Design review of the part built by this model. Coordinates are the model's own, in mm. Face numbers are marked on the shaded views. A direction names the side the tool comes from. Coordinates: 2 decimals unless noted, no trailing zeros. Write each loop counter-clockwise with the first axis right and the second up, starting at its lowest first coordinate (ties: lowest second). Pieces come first, ordered by that corner, then holes. Notation, with made-up numbers: (45, 1.5) -> (95, 1.5) arc R27 ccw to (95, 19.5) -> close; hole circle Ø4 at (43, 29). An arc over 180 degrees is marked (long way). Return JSON: item names as keys, results as strings. Group by question number.
from build123d import *

# Parameters (mm, degrees)
SKETCH_3_W          = 280
SKETCH_3_H          = 100
EXTRUDE_1_DEPTH     = 10
SKETCH_5_R          = 4
CUT_EXTRUDE_1_DEPTH = 149.996644258
SKETCH_6_R          = 4
CUT_EXTRUDE_2_DEPTH = 10
SKETCH_7_W          = 50
SKETCH_7_H          = 40
CUT_EXTRUDE_3_DEPTH = 149.996644258
FILLET_1_R          = 10
FILLET_2_R          = 10
SKETCH_8_W          = 40
SKETCH_8_H          = 40
CUT_EXTRUDE_4_DEPTH = 149.996644258
SKETCH_11_R         = 11
CUT_EXTRUDE_5_DEPTH = 5


with BuildPart() as part:
    # 草图3 → 凸台-拉伸1 (new body)
    with BuildSketch(Plane(origin=(0, 0, 0), x_dir=(1, 0, 0), z_dir=(0, 1, 0))):
        Rectangle(SKETCH_3_W, SKETCH_3_H)
    extrude(amount=EXTRUDE_1_DEPTH)

    # 草图5 → 切除-拉伸1 (cut, through all)
    with BuildSketch(Plane(origin=(0, 10, 0), x_dir=(1, 0, 0), z_dir=(0, 1, 0))):
        with Locations(Location((-115, -30, 0), (0, 0, 270))):
            Circle(SKETCH_5_R)
        with Locations(Location((-90, -30, 0), (0, 0, 270))):
            Circle(SKETCH_5_R)
    cut_extrude_1 = extrude(amount=-CUT_EXTRUDE_1_DEPTH, mode=Mode.SUBTRACT)

    # 镜向1: 切除-拉伸1 across plane
    add(cut_extrude_1.mirror(Plane.XY), mode=Mode.SUBTRACT)

    # 草图6 → 切除-拉伸2 (cut)
    with BuildSketch(Plane(origin=(0, 10, 0), x_dir=(1, 0, 0), z_dir=(0, 1, 0))):
        with Locations(Location((125, 30, 0), (0, 0, 270))):
            Circle(SKETCH_6_R)
        with Locations(Location((100, 30, 0), (0, 0, 270))):
            Circle(SKETCH_6_R)
    cut_extrude_2 = extrude(amount=-CUT_EXTRUDE_2_DEPTH, mode=Mode.SUBTRACT)

    # 镜向2: 切除-拉伸2 across plane
    add(cut_extrude_2.mirror(Plane.XY), mode=Mode.SUBTRACT)

    # 草图7 → 切除-拉伸3 (cut, through all)
    with BuildSketch(Plane(origin=(0, 10, 0), x_dir=(1, 0, 0), z_dir=(0, 1, 0))):
        with Locations((-115, 0)):
            Rectangle(SKETCH_7_W, SKETCH_7_H)
    extrude(amount=-CUT_EXTRUDE_3_DEPTH, mode=Mode.SUBTRACT)

    # 圆角1
    fillet_1_edges = [part.edges().sort_by_distance(p)[0] for p in [
        (-140, 5, 50),
    ]]
    fillet(fillet_1_edges, radius=FILLET_1_R)

    # 圆角2
    fillet_2_edges = [part.edges().sort_by_distance(p)[0] for p in [
        (-140, 5, -50),
    ]]
    fillet(fillet_2_edges, radius=FILLET_2_R)

    # 草图8 → 切除-拉伸4 (cut, through all)
    with BuildSketch(Plane(origin=(0, 10, 0), x_dir=(1, 0, 0), z_dir=(0, 1, 0))):
        with Locations((120, 0)):
            Rectangle(SKETCH_8_W, SKETCH_8_H)
    extrude(amount=-CUT_EXTRUDE_4_DEPTH, mode=Mode.SUBTRACT)

    # 草图11 → 切除-拉伸5 (cut)
    with BuildSketch(Plane(origin=(0, 10, 0), x_dir=(1, 0, 0), z_dir=(0, 1, 0))):
        with Locations(Location((-69.5, -34.5, 0), (0, 0, 270))):
            Circle(SKETCH_11_R)
        with Locations(Location((-69.5, 34.5, 0), (0, 0, 270))):
            Circle(SKETCH_11_R)
        with Locations(Location((69.5, 34.5, 0), (0, 0, 270))):
            Circle(SKETCH_11_R)
        with Locations(Location((69.5, -34.5, 0), (0, 0, 270))):
            Circle(SKETCH_11_R)
    extrude(amount=-CUT_EXTRUDE_5_DEPTH, mode=Mode.SUBTRACT)


solid = part.part
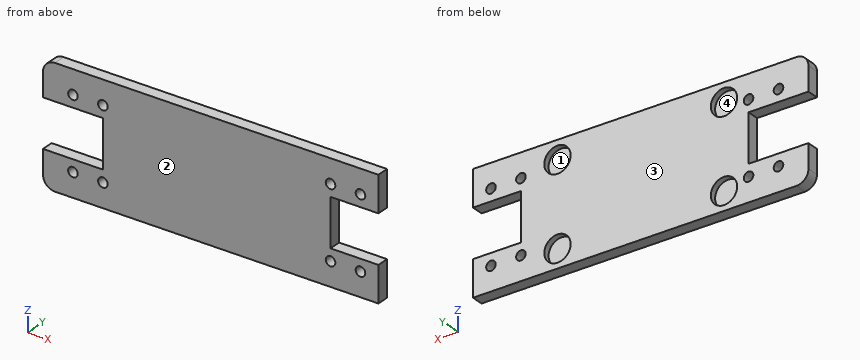
Q1. Wall thickness on L1, parallel to X at y = 7.7, z = -34.5; L2, parallel to X at y = 4, z = -30; L3, parallel to Z at x = -118, y = 1: over which ranges is each line inside the solid? List them lowest first.
Q2. We need section A-A on y = 2.5. State how many separate pieces and enclosed holes the cut face has, plus the area to 3 significant figures.
Q3. For the marked faces 3 and 4, list the 3-axis set-ups (+Z, -Z, +X, -X, +Y, -Y) from which the entire face can be reached by the end or side of a thin tool; tool diameter is ignored.
Q4. The part is to be moulded in two halves that separate along X. For the marked faces 1 and 2, say which applies: +X half, -X half, draft (parallel to the pull), parting line (faces both ways), or undercut.
Q5. For P1, Ø4, axis at y = 4, z = 12.5, coming from the -X side; P2, Ø2, axis at x = -77, z = 28.5, coming from the +Y side, all flat-tipped, find the tip position at first contact; note any pin that passes through.
Q6. We need section C-C on x = -69.5. Write out the cut boundary in (y, z).
Q7. We need section B-B on z = 30. Write out the cut boundary in (x, y).
Findings below:
{
 "1": {"L1": "x = -140 to -80.5, -58.5 to 58.5, 80.5 to 140", "L2": "x = -140 to -119, -111 to -94, -86 to 96, 104 to 121, 129 to 140", "L3": "z = -50 to -32.65, -27.35 to -20, 20 to 27.35, 32.65 to 50"},
 "2": {"separate pieces": "1", "enclosed holes": "8", "area": "24,000 mm^2"},
 "3": {"face 3": "+Z, -Z, +X, -X, +Y", "face 4": "+Y"},
 "4": {"face 1": "undercut", "face 2": "draft"},
 "5": {"P1": "stops at x = -90", "P2": "stops at y = 5"},
 "6": {"outline": "(0, -50) -> (10, -50) -> (10, -45.5) -> (5, -45.5) -> (5, -23.5) -> (10, -23.5) -> (10, 23.5) -> (5, 23.5) -> (5, 45.5) -> (10, 45.5) -> (10, 50) -> (0, 50) -> close"},
 "7": {"outline": "(-140, 0) -> (-119, 0) -> (-119, 10) -> (-140, 10) -> close; (-111, 0) -> (-94, 0) -> (-94, 10) -> (-111, 10) -> close; (-86, 0) -> (96, 0) -> (96, 10) -> (79.54, 10) -> (79.54, 5) -> (59.46, 5) -> (59.46, 10) -> (-59.46, 10) -> (-59.46, 5) -> (-79.54, 5) -> (-79.54, 10) -> (-86, 10) -> close; (104, 0) -> (121, 0) -> (121, 10) -> (104, 10) -> close; (129, 0) -> (140, 0) -> (140, 10) -> (129, 10) -> close"}
}
